The drawing under review shows one solid part. Ordinate dimensions are in mm from its lowest x, y, z. A direction names the side the tool comes from. Coordinates: 2 decimals unless noted, no trailing zeros. Write each loop counter-clockwise with the first axis right and the second up, starting at its lowest first coordinate (ties: lowest second). Pieces come first, ordered by that corner, then holes.
1) Add section B-B, the plane z = 11. State the section outline as (x, y) points, then the cut area to 3 significant figures.
2) Mouldability with a two-part tool opening along Y and no side actions: class the marked faces 1, 2, 3 and 4 as released by +Y, released by -Y, zero draft, split by the parting line, or undercut.
3) For P1, Ø2, axis at y = 56, z = 28, coming from the -X side; P2, Ø1.5, axis at x = 28.5, z = 24, coming from the +Y side; P3, Ø5, axis at y = 26, z = 10.5, coming from the +X side; P4, Ø8, axis at x = 31.5, y = 7.5, coming from the +Z side, all flat-tipped, find the tip position at first contact; note any pin that passes through.
4) For line 1 (Y direction, x = 11.5, z = 19.5); line 2 (X direction, y = 40, z = 6); line 3 (Y direction, x = 44.5, z = 32.5), list the stretches that pass through material, from the lowest coordinate up.
5) Add section C-C, the plane y = 8. State the section outline as (x, z) points, then the cut area to 3 significant figures.
6) Add section A-A, the plane x = 39.5. State the section outline as (y, z) points, then the cut area to 3 significant figures.
7) Machinability: for the marked faces 5, 6 and 7, which of the approach directions +Z, -Z, +X, -X, +Y, -Y give a long, thin tool a straight path to every point of the face, cutting with its end or side? Answer none if there is none.
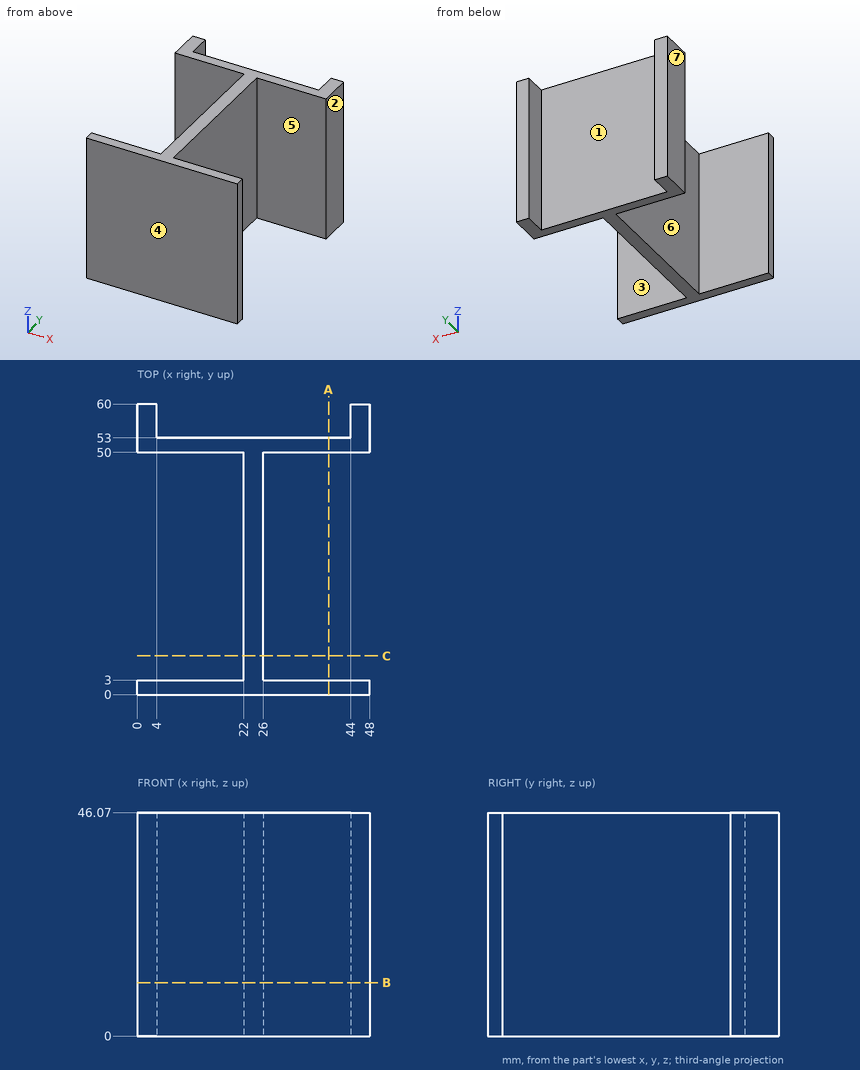
Geometry results:
1. outline: (0, 0) - (48, 0) - (48, 3) - (26, 3) - (26, 50) - (48, 50) - (48, 60) - (44, 60) - (44, 53) - (4, 53) - (4, 60) - (0, 60) - (0, 50) - (22, 50) - (22, 3) - (0, 3) - close
1. area: 532 mm2
2. face 1: released by +Y
2. face 2: zero draft
2. face 3: undercut
2. face 4: released by -Y
3. P1: stops at x = 0
3. P2: stops at y = 53
3. P3: stops at x = 26
3. P4: passes through
4. line 1: y = 0 to 3, 50 to 53
4. line 2: x = 22 to 26
4. line 3: y = 0 to 3, 50 to 60
5. outline: (22, 0) - (26, 0) - (26, 46.07) - (22, 46.07) - close
5. area: 184 mm2
6. outline: (0, 0) - (3, 0) - (3, 46.07) - (0, 46.07) - close; (50, 0) - (53, 0) - (53, 46.07) - (50, 46.07) - close
6. area: 276 mm2
7. face 5: +Z, -Z, +X
7. face 6: +Z, -Z, -X
7. face 7: +Z, -Z, -X, +Y, -Y
